Design review of the part built by this model. Coordinates are the model's own, in mm. Face numbers are marked on the shaded views. A direction names the side the tool comes from. Coordinates: 2 decimals unless noted, no trailing zeros. Write each loop counter-clockwise with the first axis right and the second up, starting at its lowest first coordinate (ties: lowest second). Pieces come first, ordered by that corner, then holes.
Q1. For probe 1 along Y at (x, z) = (0, -6.5); probe 2 along X at (y, z) = (2.25, -2); probe 3 along Y at (x, z) = (-1.5, 3.25), list the stretches that pass through material, from the lowest coordinate up.
Q2. Take a section at C-C (z = -8). Give the boundary of the cut face in (x, y), and give its area (3 significant figures).
Q3. Insertion check: pin 1 (5 mm diameter, centred on x = -3, z = -7, fed in from -Y); pin 2 (6 mm diameter, centred on y = 4, z = 8.5, fed in from -X); pin 3 (4 mm diameter, centred on x = 2, y = -3.5, fed in from -Z); pin 4 (4 mm diameter, centred on x = -2.5, z = -9, fed in from +Y). Each pin has a flat end and moves straight along its axis. Give the tip position at first contact, or say it passes through.
Q4. Take a section at A-A (z = 1). Give the boundary of the cut face in (x, y), and give its area (3 significant figures).
Q5. Take a section at B-B (x = 0). Give the boundary of the cut face in (y, z), and give its area (3 significant figures).
Q6. Machinability: for the marked faces 1, 2 and 3, which of the approach directions +Z, -Z, +X, -X, +Y, -Y give a long, thin tool a straight path to every point of the face, cutting with its end or side? Answer none if there is none.
```python
from build123d import *

# Parameters (mm, degrees)
BOSS_EXTRUDE1_DEPTH = 3
SKETCH2_R           = 4.5
BOSS_EXTRUDE2_DEPTH = 9.4
SKETCH3_R           = 2.6
CUT_EXTRUDE1_DEPTH  = 15.978095117
CHAMFER2_SIZE       = 0.7


# Read off the part's stored shape, not the designer's step: Mirror3
with BuildPart() as part:
    # Sketch1 → Boss-Extrude1 (new body)
    with BuildSketch(Plane.XY):
        Polygon((6.350852961, 0), (3.175426481, 5.5), (-3.175426481, 5.5), (-6.350852961, 0), (-3.175426481, -5.5), (3.175426481, -5.5), align=None)
    extrude(amount=BOSS_EXTRUDE1_DEPTH)

    # Sketch2 → Boss-Extrude2 (add)
    with BuildSketch(Plane.XY.offset(3)):
        Circle(SKETCH2_R)
    extrude(amount=BOSS_EXTRUDE2_DEPTH)

    # Sketch3 → Cut-Extrude1 (cut, through all)
    with BuildSketch(Plane(origin=(0, 0, 0), x_dir=(-1, 0, 0), z_dir=(0, 0, -1))):
        Circle(SKETCH3_R)
    extrude(amount=-CUT_EXTRUDE1_DEPTH, mode=Mode.SUBTRACT)

    # Sketch5 → Cut-Revolve2 (revolve, cut)
    with BuildSketch(Plane(origin=(0, 0, 0), x_dir=(1, 0, 0), z_dir=(0, 1, 0)), mode=Mode.PRIVATE) as cut_revolve2_sk:
        Polygon((-4.5, -3), (-6.350852961, -3), (-6.350852961, -2.5), align=None)
    revolve(cut_revolve2_sk.sketch.rotate(Axis((0, 0, 12.4), (0, 0, -1)), 180), axis=Axis((0, 0, 12.4), (0, 0, -1)), mode=Mode.SUBTRACT)

    # Mirror3: part across plane


with BuildPart() as part_1:
    add(part.part)
    add(part.part.mirror(Plane.XY))

    # Chamfer2
    chamfer2_edges = [part_1.edges().sort_by_distance(p)[0] for p in [
        (-4.5, 0, 12.4),
        (-4.5, 0, -12.4),
    ]]
    chamfer(chamfer2_edges, length=CHAMFER2_SIZE)


solid = part_1.part
```
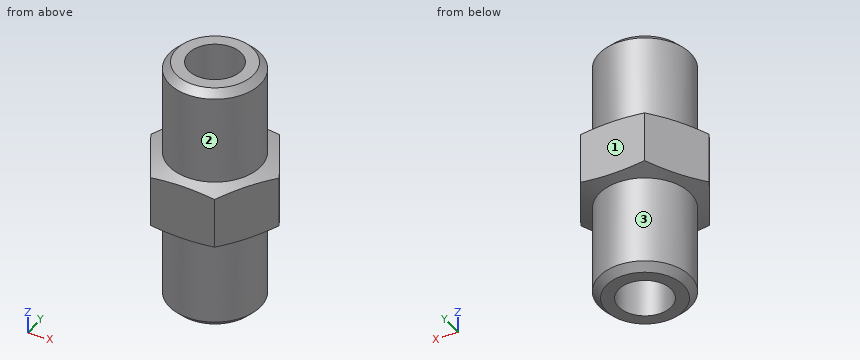
Response:
1. probe 1: y = -4.5 to -2.6, 2.6 to 4.5
1. probe 2: x = -5.05 to -1.3, 1.3 to 5.05
1. probe 3: y = -4.24 to -2.12, 2.12 to 4.24
2. outline: circle Ø9 at (0, 0); hole circle Ø5.2 at (0, 0)
2. area: 42.4 mm2
3. pin 1: stops at y = -4.47
3. pin 2: stops at x = -4.39
3. pin 3: stops at z = -12.4
3. pin 4: stops at y = 4.47
4. outline: (-6.35, 0) - (-3.18, -5.5) - (3.18, -5.5) - (6.35, 0) - (3.18, 5.5) - (-3.18, 5.5) - close; hole circle Ø5.2 at (0, 0)
4. area: 83.6 mm2
5. outline: (-5.5, -2.73) - (-4.5, -3) - (-4.5, -11.7) - (-3.8, -12.4) - (-2.6, -12.4) - (-2.6, 12.4) - (-3.8, 12.4) - (-4.5, 11.7) - (-4.5, 3) - (-5.5, 2.73) - close; (2.6, -12.4) - (3.8, -12.4) - (4.5, -11.7) - (4.5, -3) - (5.5, -2.73) - (5.5, 2.73) - (4.5, 3) - (4.5, 11.7) - (3.8, 12.4) - (2.6, 12.4) - close
5. area: 105 mm2
6. face 1: +Z, -Z, +X, -X, +Y
6. face 2: +Z
6. face 3: -Z
